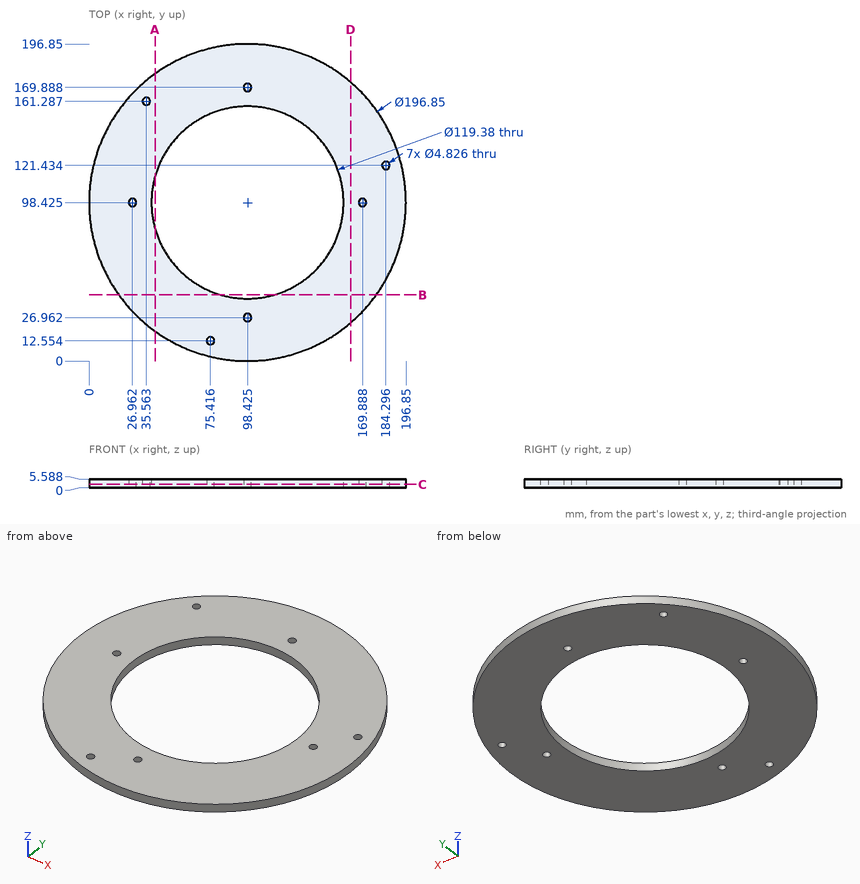
Check sheet for the drawn part. Datum: minimum x, y, z corner. Units: mm. Round coordinates to 2 decimals unless told otherwise and drop trailing zeros. Loops run counter-clockwise (first coordinate to the right, second up) from the corner with the lowest first, then second, coordinate; pieces in that order, holes last. Notation, with made-up numbers: (-27, 51) - (22, 51) arc R14 cw to (22, 62) - close; hole circle Ø5 at (68, -28.5). An arc over 180 degrees is marked (long way). Answer as a JSON object with one key per item and string values. Group by question number.
Q1. Gauge pin test, flat ends, axial feed: P1, Ø1, axis at x = 100.5, z = 3.5, coming from the -Y side; P2, Ø4.5, axis at x = 35.56, y = 161.29, coming from the +Z side; P3, Ø1.5, axis at y = 107, z = 4, coming from the +X side; P4, Ø3, axis at x = 123, z = 3.5, coming from the +Y side. Record the tip position at first contact, or that the pin passes through.
Q2. Sectioned sample at D-D, the plane x = 162.5. Enter the section's corners in (y, z), plus the area to 3 significant figures.
Q3. Sectioned sample at C-C, the plane z = 2.3. Count the separate pieces of the cut face and the enclosed holes in it, plus the area to 3 significant figures.
Q4. Sectioned sample at A-A, the plane x = 41. Enter the section's corners in (y, z), plus the area to 3 significant figures.
Q5. Scan lines: line 1 along Y through (x, z) = (98, 4.8); line 2 along X through (y, z) = (100, 5) (1 decimal); line 3 along Y through (x, z) = (163.5, 5). Record each from-to range of solid material in increasing order. Write a range as [from, to].
Solution:
{
 "1": {"P1": "stops at y = 0.01", "P2": "passes through", "P3": "stops at x = 196.54", "P4": "stops at y = 194.11"},
 "2": {"outline": "(23.71, 0) - (173.14, 0) - (173.14, 5.59) - (23.71, 5.59) - close", "area": "835 mm²"},
 "3": {"separate pieces": "1", "enclosed holes": "8", "area": "19,100 mm²"},
 "4": {"outline": "(18.49, 0) - (82.14, 0) - (82.14, 5.59) - (18.49, 5.59) - close; (114.71, 0) - (178.36, 0) - (178.36, 5.59) - (114.71, 5.59) - close", "area": "711 mm²"},
 "5": {"line 1": "y = [0, 24.59], [29.34, 38.74], [158.11, 167.51], [172.26, 196.85]", "line 2": "x = [0, 25.1], [28.8, 38.8], [158.1, 168.1], [171.7, 196.8]", "line 3": "y = [24.58, 172.27]"}
}
